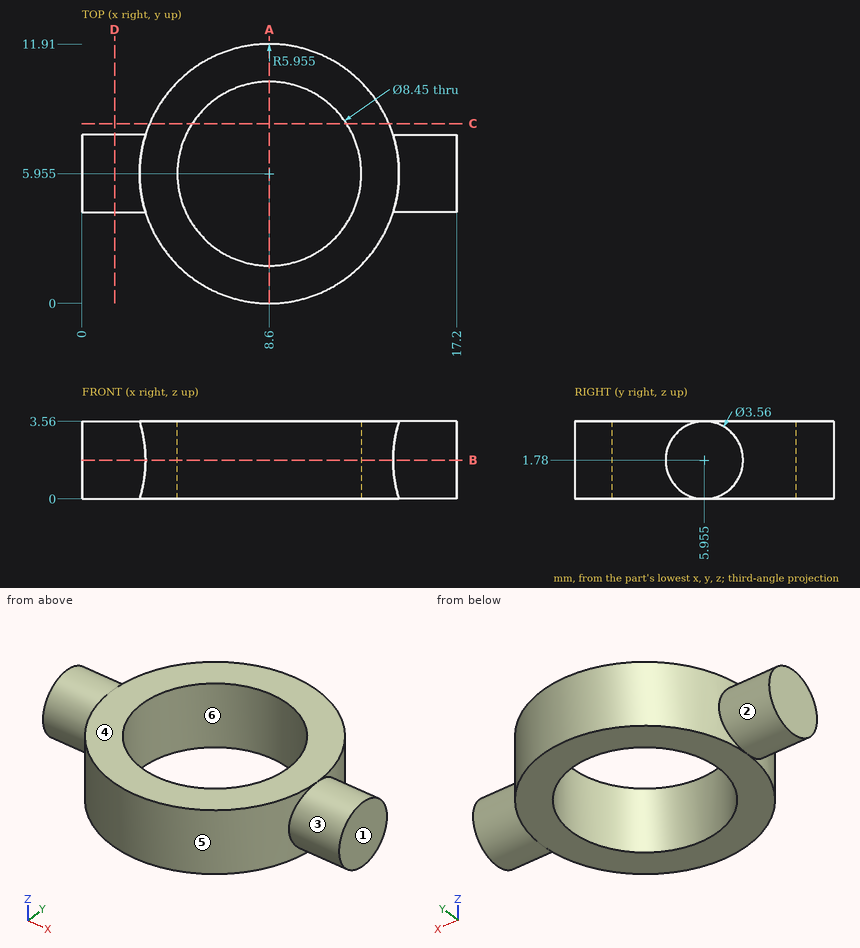
Study the drawing (mm; zero at the part's minimum x, y, z) and answer. A direction names the side the tool comes from. Give positions to 0.01 mm unless a question says otherwise; leave off trailing zeros. Loops run counter-clockwise (first coordinate to the right, second up) from the corner with the lowest first, then second, coordinate; pieces in that order, holes last. Notation, with made-up numbers: (42, -12) - (83, -12) arc R30 ccw to (83, 15) - close; hole circle Ø9 at (58.5, 87). An arc over 180 degrees is marked (long way). Return JSON: item names as keys, results as strings. Group by question number.
1. Find section C-C (y = 8.25). Write down the section's boundary in (x, z) (3 decimals), then the cut area to 3 significant figures.
2. Find section D-D (x = 1.5). Write down the section's boundary in (y, z) (3 decimals), then the cut area to 3 significant figures.
3. Find section B-B (z = 1.78). Write down the section's boundary in (x, y) (3 decimals).
4. Determine the mould class of the marked faces 4, 5 and 6 for opening direction Y: pulls with the +Y half, pulls with the -Y half, needs draft (parallel to the pull), parting line crosses it, or undercut.
5. Given pin 1 Ø3 at (x, y) = (6.5, 4) entering from +Z, flat-ended and moving along its own axis, determine where the tip first touches the part or whether it passes through.
6. Find section A-A (x = 8.6). Write down the section's boundary in (y, z).
7. Which of the six approach directions +Z, -Z, +X, -X, +Y, -Y give full straight-line access (tool end or side, diameter ignored) to the marked faces 1, 2 and 3?
8. Straight lines are drawn through the part: line 1 (Y direction, x = 8.6, z = 2.85); line 2 (X direction, y = 6, z = 1.6); line 3 (X direction, y = 9.75, z = 1.75). For each, find the intervals that lie inside material, in ascending order. Write a range as [from, to].
Verdict:
{
 "1": {"outline": "(3.105, 0) - (5.053, 0) - (5.053, 3.56) - (3.105, 3.56) - close; (12.147, 0) - (14.095, 0) - (14.095, 3.56) - (12.147, 3.56) - close", "area": "13.9 mm^2"},
 "2": {"outline": "circle Ø3.56 at (5.955, 1.78)", "area": "9.95 mm^2"},
 "3": {"outline": "(0, 4.175) - (2.917, 4.175) arc R5.955 ccw to (14.283, 4.175) - (17.2, 4.175) - (17.2, 7.735) - (14.283, 7.735) arc R5.955 ccw to (2.917, 7.735) - (0, 7.735) - close; hole circle Ø8.45 at (8.6, 5.955)"},
 "4": {"face 4": "needs draft", "face 5": "pulls with the -Y half", "face 6": "undercut"},
 "5": {"pin 1": "stops at z = 3.56"},
 "6": {"outline": "(0, 0) - (1.73, 0) - (1.73, 3.56) - (0, 3.56) - close; (10.18, 0) - (11.91, 0) - (11.91, 3.56) - (10.18, 3.56) - close"},
 "7": {"face 1": "+Z, -Z, +X, +Y, -Y", "face 2": "-X", "face 3": "+X"},
 "8": {"line 1": "y = [0, 1.73], [10.18, 11.91]", "line 2": "x = [0, 4.38], [12.82, 17.2]", "line 3": "x = [4.01, 6.74], [10.46, 13.19]"}
}
